Here's how the part is built. I have some questions about the finished solid (model axes, mm). Face numbers are marked on the shaded views. Round coordinates to 2 decimals unless told otherwise and drop trailing zeros. Order: outer loops, then holes, each group sorted by start corner. A loop starts at its lowest first (then second) coordinate and runs counter-clockwise, first axis right, second up. Notation, with made-up numbers: M -15.75,-17.5 L 24.25,-17.5 A10 cw 24.25,-1.5 Z; hole C 40.5,63.25 d5. An arc over 180 degrees is marked long. Write each question's results on one line, items separated by ' | '. Start each with the question number.
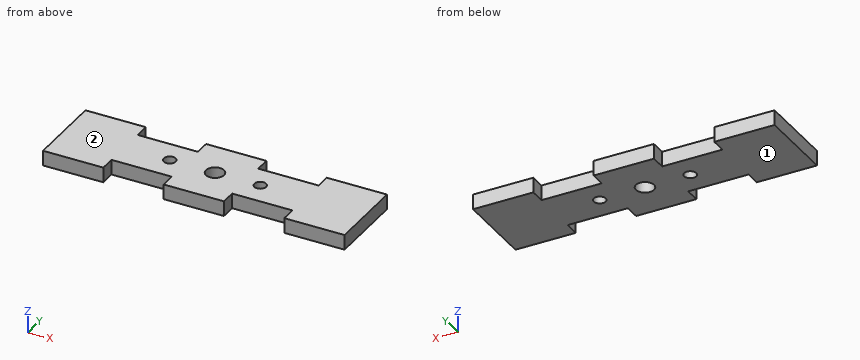
```python
from build123d import *

# Parameters (mm, degrees)
CROQUIS1_R              = 1.5
CROQUIS1_R_2            = 0.977820283
CROQUIS1_R_3            = 1
SALIENTE_EXTRUIR1_DEPTH = 2.5


with BuildPart() as part:
    # Croquis1 → Saliente-Extruir1 (new body)
    with BuildSketch(Plane.XY):
        Polygon((-25, 6.5), (-15, 6.5), (-15, 4), (-5, 4), (-5, 6.5), (5, 6.5), (5, 4), (15, 4), (15, 6.5), (25, 6.5), (25, -6.5), (15, -6.5), (15, -4), (5, -4), (5, -6.5), (-5, -6.5), (-5, -4), (-15, -4), (-15, -6.5), (-25, -6.5), align=None)
        Circle(CROQUIS1_R, mode=Mode.SUBTRACT)
        with Locations((7.5, 0)):
            Circle(CROQUIS1_R_2, mode=Mode.SUBTRACT)
        with Locations((-7.5, 0)):
            Circle(CROQUIS1_R_3, mode=Mode.SUBTRACT)
    extrude(amount=SALIENTE_EXTRUIR1_DEPTH)


solid = part.part
```
(1) I want a section at C-C on z = 1.05. Write out the boundary of the cut face in (x, y), and give its area (3 significant figures).
(2) Please list where these lines run through material, in increasing order: line 1 (X direction, y = -6, z = 1.5); line 2 (Y direction, x = -7.5, z = 0.9); line 3 (Y direction, x = 0, z = 2).
(3) If we mould it in two halves opening along Z, with no side actions, what happens to the marked faces 1 and 2? For each: pulls with the +Z half, pulls with the -Z half, needs draft (parallel to the pull), parting line crosses it, or undercut.
(4) I want a section at A-A on y = 0. Write out the boundary of the cut face in (x, z), and give its area (3 significant figures).
(5) I want a section at B-B on x = 0. Write out the boundary of the cut face in (y, z), and give its area (3 significant figures).
(6) I'm going to push flat-ended pins straight in: pin 1 Ø1.2 at (x, z) = (9.5, 2) entering from +Y; pin 2 Ø1 at (x, z) = (-9, 1.5) entering from -Y. Where does each tip first touch, or does it pass through?
(7) I want a section at D-D on x = 7.5. Write out the boundary of the cut face in (y, z), and give its area (3 significant figures).
Solutions:
1) outline: M -25,-6.5 L -15,-6.5 L -15,-4 L -5,-4 L -5,-6.5 L 5,-6.5 L 5,-4 L 15,-4 L 15,-6.5 L 25,-6.5 L 25,6.5 L 15,6.5 L 15,4 L 5,4 L 5,6.5 L -5,6.5 L -5,4 L -15,4 L -15,6.5 L -25,6.5 Z; hole C -7.5,0 d2; hole C 0,0 d3; hole C 7.5,0 d1.96 | area: 537 mm^2
2) line 1: -25 to -15, -5 to 5, 15 to 25 | line 2: -4 to -1, 1 to 4 | line 3: -6.5 to -1.5, 1.5 to 6.5
3) face 1: pulls with the -Z half | face 2: pulls with the +Z half
4) outline: M -25,0 L -8.5,0 L -8.5,2.5 L -25,2.5 Z; M -6.5,0 L -1.5,0 L -1.5,2.5 L -6.5,2.5 Z; M 1.5,0 L 6.52,0 L 6.52,2.5 L 1.5,2.5 Z; M 8.48,0 L 25,0 L 25,2.5 L 8.48,2.5 Z | area: 108 mm^2
5) outline: M -6.5,0 L -1.5,0 L -1.5,2.5 L -6.5,2.5 Z; M 1.5,0 L 6.5,0 L 6.5,2.5 L 1.5,2.5 Z | area: 25.0 mm^2
6) pin 1: y = 4 | pin 2: y = -4
7) outline: M -4,0 L -0.98,0 L -0.98,2.5 L -4,2.5 Z; M 0.98,0 L 4,0 L 4,2.5 L 0.98,2.5 Z | area: 15.1 mm^2
